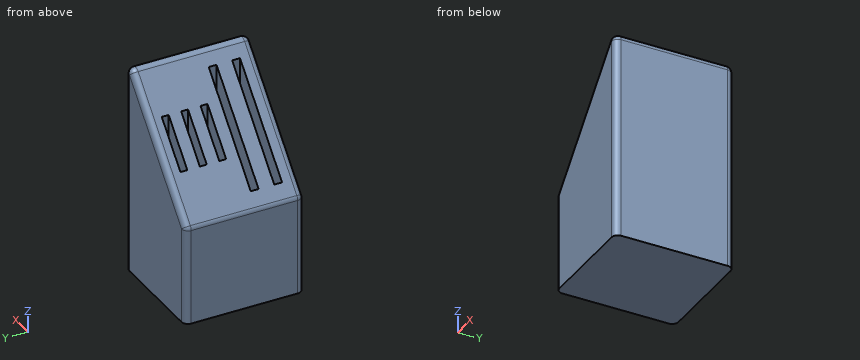
```python
from build123d import *

# Parameters (mm, degrees)
F1_DEPTH = 38
F3_W     = 25
F3_H     = 2.5
F4_DEPTH = 45
F3_W_2   = 11.1
F3_H_2   = 2.2
F5_DEPTH = 30.5
F6_R     = 2


with BuildPart() as f1:
    # F0 (on Front) → F1 (new body)
    with BuildSketch(Plane.XZ):
        Polygon((0, -31.542231), (0, 38.457769), (-35, 0), (-35, -31.542231), align=None)
    extrude(amount=F1_DEPTH)

    # F3 (on offset) → F4 (cut)
    with BuildSketch(Plane.XY.offset(39)):
        with Locations((-18.802461, -31.75)):
            Rectangle(F3_W, F3_H)
        with Locations((-18.802461, -24.25)):
            Rectangle(F3_W, F3_H)
    extrude(amount=-F4_DEPTH, mode=Mode.SUBTRACT)

    # F3 (on offset) → F5 (cut)
    with BuildSketch(Plane.XY.offset(39)):
        with Locations((-18.576984, -11.7)):
            Rectangle(F3_W_2, F3_H_2)
        with Locations((-18.576984, -17.9)):
            Rectangle(F3_W_2, F3_H_2)
        with Locations((-18.576984, -5.5)):
            Rectangle(F3_W_2, F3_H_2)
    extrude(amount=-F5_DEPTH, mode=Mode.SUBTRACT)

    # F6
    f6_edges = [f1.edges().sort_by_distance(p)[0] for p in [
        (-17.5, 0, 19.228885),
        (-35, -19, 0),
        (-17.5, -38, 19.228885),
        (0, -19, 38.457769),
        (0, 0, 3.457769),
        (0, -38, 3.457769),
        (-35, 0, -15.771115),
        (-35, -38, -15.771115),
    ]]
    fillet(f6_edges, radius=F6_R)


solid = f1.part
```
Verification items for the finished model (mm, model axes). Round coordinates to 2 decimals unless told otherwise and drop trailing zeros. Order: outer loops, then holes, each group sorted by start corner. A loop starts at its lowest first (then second) coordinate and runs counter-clockwise, first axis right, second up.
1) Material ranges on line 1 (Y direction, x = -8, z = 24.5); line 2 (Y direction, x = -9, z = 28); line 3 (Z direction, x = -9, y = -31.5), recorded low to high.
Geometry says:
line 1: y = -38 to -33, -30.5 to -25.5, -23 to 0
line 2: y = -37.18 to -33, -30.5 to -25.5, -23 to -0.82
line 3: z = -31.54 to -6
2) Cross-section at A-A, the plane y = -24.5. Record the cut outline in (x, z), plus the area to 3 significant figures.
Geometry says:
outline: (-35, -31.54) - (0, -31.54) - (0, 33.29) arc R2 ccw to (-3.48, 34.63) - (-6.3, 31.53) - (-6.3, -6) - (-31.3, -6) - (-31.3, 4.06) - (-34.48, 0.57) arc R2 ccw to (-35, -0.77) - close
area: 1,180 mm2
3) Cross-section at C-C, the plane z = 10. Give the number of separate pieces and of enclosed holes in the cut face, plus the area to 3 significant figures.
Geometry says:
separate pieces: 1
enclosed holes: 3
area: 809 mm2
4) Depth check by flat-ended pin: pin 1 (2 mm diameter, centred on x = -13, y = -32.5, fed in from +Z); pin 2 (2.5 mm diameter, centred on y = -6, z = 13.5, fed in from -X); pin 3 (3 mm diameter, centred on y = -32, z = 9, fed in from -X). Enter the tip coordinate at first touch or a pass-through.
Geometry says:
pin 1: stops at z = 25.13
pin 2: stops at x = -23.71
pin 3: stops at x = -27.83
5) Cross-section at B-B, the plane y = -11.5. Record the cut outline in (x, z).
Geometry says:
outline: (-35, -31.54) - (0, -31.54) - (0, 33.29) arc R2 ccw to (-3.48, 34.63) - (-13.03, 24.14) - (-13.03, 8.5) - (-24.13, 8.5) - (-24.13, 11.95) - (-34.48, 0.57) arc R2 ccw to (-35, -0.77) - close
